from build123d import *

# Parameters (mm, degrees)
SKETCH1_R           = 1.4224
BOSS_EXTRUDE1_DEPTH = 6.35
SKETCH2_R           = 2.7051
BOSS_EXTRUDE2_DEPTH = 1.4986
FILLET1_R           = 1.016
CUT_EXTRUDE1_DEPTH  = 2.38125


with BuildPart() as part:
    # Sketch1 → Boss-Extrude1 (new body)
    with BuildSketch(Plane(origin=(0, 0, 0), x_dir=(1, 0, 0), z_dir=(0, 1, 0))):
        Circle(SKETCH1_R)
    extrude(amount=BOSS_EXTRUDE1_DEPTH)

    # Sketch2 → Boss-Extrude2 (add)
    with BuildSketch(Plane(origin=(0, 6.35, 0), x_dir=(1, 0, 0), z_dir=(0, 1, 0))):
        Circle(SKETCH2_R)
    extrude(amount=BOSS_EXTRUDE2_DEPTH)

    # Fillet1
    fillet1_edges = [part.edges().sort_by_distance(p)[0] for p in [
        (-2.7051, 7.8486, 0),
    ]]
    fillet(fillet1_edges, radius=FILLET1_R)

    # Sketch3 → Cut-Extrude1 (cut)
    with BuildSketch(Plane(origin=(0, 7.8486, 0), x_dir=(1, 0, 0), z_dir=(0, 1, 0))):
        Polygon((0, 0.916543552), (-0.79375, 0.458271776), (-0.79375, -0.458271776), (0, -0.916543552), (0.79375, -0.458271776), (0.79375, 0.458271776), align=None)
    extrude(amount=-CUT_EXTRUDE1_DEPTH, mode=Mode.SUBTRACT)


solid = part.part
The model under review builds one solid part; all positions refer to its coordinate system, in mm. A direction names the side the tool comes from. Coordinates: 2 decimals unless noted, no trailing zeros. Write each loop counter-clockwise with the first axis right and the second up, starting at its lowest first coordinate (ties: lowest second). Pieces come first, ordered by that corner, then holes. Notation, with made-up numbers: (-23, -31.75) - (19, -31.75) arc R3 cw to (19, -27.75) - close; hole circle Ø8 at (6, 54). An arc over 180 degrees is marked (long way). Answer as CSV lines item,"result".
(1) For line 1 along Y through (x, z) = (0, 0.75); line 2 along X through (y, z) = (7, -0.2); line 3 along Z through (x, y) = (-0.05, 6.5), list the stretches that pass through material, from the lowest coordinate up. Write a range as [from, to].
Data:
line 1,"y = [0, 5.47]"
line 2,"x = [-2.68, -0.79], [0.79, 2.68]"
line 3,"z = [-2.7, -0.89], [0.89, 2.7]"
(2) Clearance check with flat-ended pins moving along their axes: pin 1 Ø1 at (x, z) = (-1.5, 1.5) entering from -Y; pin 2 Ø1 at (x, y) = (-1.5, 2.5) entering from -Z. State where each tip first meets the part, or that it passes through.
Data:
pin 1,"stops at y = 6.35"
pin 2,"stops at z = -1.01"
(3) We need section A-A (y = 6.5). Give the boundary of the cut face in (x, z).
Data:
outline,"circle Ø5.41 at (0, 0); hole (-0.79, -0.46) - (0, -0.92) - (0.79, -0.46) - (0.79, 0.46) - (0, 0.92) - (-0.79, 0.46) - close"
(4) We need section B-B (z = 0). Give the boundary of the cut face in (x, y).
Data:
outline,"(-2.71, 6.35) - (-1.42, 6.35) - (-1.42, 0) - (1.42, 0) - (1.42, 6.35) - (2.71, 6.35) - (2.71, 6.83) arc R1.02 ccw to (1.69, 7.85) - (0.79, 7.85) - (0.79, 5.47) - (-0.79, 5.47) - (-0.79, 7.85) - (-1.69, 7.85) arc R1.02 ccw to (-2.71, 6.83) - close"
(5) Tool access review of faces 4 (the flat face through (1.2, 6.35, 1.2)), 5 (the cylindrical face through (2.58, 6.59, -0.81)), 6 (the flat face through (0.794, 7, 0)): name each direction out of +Z, -Z, +X, -X, +Y, -Y from which nothing blocks a thin tool from reaching the whole face with its end or side.
Data:
face 4,"-Y"
face 5,"+Y, -Y"
face 6,"+Y"
(6) We need section C-C (y = 4.5). Give the boundary of the cut face in (x, z).
Data:
outline,"circle Ø2.84 at (0, 0)"
(7) Mouldability with a two-part tool opening along Z and no side actions: class faces 1 (the cylindrical face through (-0.31, 3.13, 1.39)), 2 (the flat face through (1, 7.849, 1)), 3 (the flat face through (-0.794, 7, 0)) as pulls with the +Z half, pulls with the -Z half, needs draft (parallel to the pull), parting line crosses it, or undercut.
Data:
face 1,"parting line crosses it"
face 2,"needs draft"
face 3,"undercut"
